from build123d import *

# Parameters (mm, degrees)
BOSS_EXTRUDE1_DEPTH       = 30
BOSS_EXTRUDE2_DEPTH       = 105
FILLET1_R                 = 5
CONVERT_SOLID2_START      = -80
CONVERT_SOLID2_DEPTH      = 160
SKETCH12_R                = 7
SKETCH12_R_2              = 2.5
AXLE_HOLES_DEPTH          = 141.121375957
SKETCH13_W                = 39.25
SKETCH13_H                = 43.333333333
SKETCH13_H_2              = 43.333333334
WEIGHT_SAVING_HOLES_DEPTH = 2
CHAMFER1_SIZE             = 5
M3_START                  = -52.5
M3_CLEARANCE_SLOT1_DEPTH  = 105
M2_CLEARANCE_HOLE1_D      = 2.4


# Read off the part's stored shape, not the designer's step: Convert-Solid2, M3 Clearance Slot1
with BuildPart() as part:
    # Sketch1 → Boss-Extrude1 (new body)
    with BuildSketch(Plane(origin=(0, 0, 0), x_dir=(1, 0, 0), z_dir=(0, 1, 0))):
        Polygon((-52.5, -80), (0, -80), (52.5, -80), (52.5, 80), (-52.5, 80), align=None)
    extrude(amount=BOSS_EXTRUDE1_DEPTH)

    # Sketch11 → Boss-Extrude2 (add)
    with BuildSketch(Plane(origin=(52.5, 0, 0), x_dir=(0, 0, -1), z_dir=(1, 0, 0))):
        with BuildLine():
            Line((-18.091022132, 30), (-15.974774553, 35.814342437))
            ThreePointArc((-15.974774553, 35.814342437), (0, 47), (15.974774553, 35.814342437))
            Line((15.974774553, 35.814342437), (18.091022132, 30))
            Line((18.091022132, 30), (-18.091022132, 30))
        make_face()
    extrude(amount=-BOSS_EXTRUDE2_DEPTH)

    # Fillet1
    fillet1_edges = [part.edges().sort_by_distance(p)[0] for p in [
        (0, 30, -18.091022132),
        (0, 30, 18.091022132),
    ]]
    fillet(fillet1_edges, radius=FILLET1_R)

    # Convert-Solid2 outline → Convert-Solid2 (cut)
    with BuildSketch(Plane.XY.offset(CONVERT_SOLID2_START)):
        with BuildLine():
            Line((-54, 5.2e-08), (-49.5, 0))
            ThreePointArc((-49.5, 0), (-51.621320344, 0.878679656), (-52.5, 3))
            Line((-52.5, 3), (-52.499999977, 48))
            Line((-52.499999977, 48), (-54, 48))
            Line((-54, 48), (-54, 5.2e-08))
        make_face()
        with BuildLine():
            ThreePointArc((52.5, 3), (51.621320344, 0.878679656), (49.5, 0))
            Line((49.5, 0), (54, 5.2e-08))
            Line((54, 5.2e-08), (54, 48))
            Line((54, 48), (52.499999977, 48))
            Line((52.499999977, 48), (52.5, 3))
        make_face()
        with BuildLine():
            Line((50.5, 3), (50.5, 48))
            Line((50.5, 48), (-50.5, 48))
            Line((-50.5, 48), (-50.5, 3))
            ThreePointArc((-50.5, 3), (-50.207106781, 2.292893219), (-49.5, 2))
            Line((-49.5, 2), (49.5, 2))
            ThreePointArc((49.5, 2), (50.207106781, 2.292893219), (50.5, 3))
        make_face()
    extrude(amount=CONVERT_SOLID2_DEPTH, mode=Mode.SUBTRACT)

    # Sketch12 → Axle Holes (cut, through all)
    with BuildSketch(Plane(origin=(52.5, 0, 0), x_dir=(0, 0, -1), z_dir=(1, 0, 0))):
        with Locations((0, 30)):
            Circle(SKETCH12_R)
        with Locations((35, 15)):
            Circle(SKETCH12_R_2)
        with BuildLine():
            Line((-35, 19.5), (-25, 19.5))
            ThreePointArc((-25, 19.5), (-22, 16.5), (-25, 13.5))
            Line((-25, 13.5), (-35, 13.5))
            ThreePointArc((-35, 13.5), (-38, 16.5), (-35, 19.5))
        make_face()
    extrude(amount=-AXLE_HOLES_DEPTH, mode=Mode.SUBTRACT)

    # Sketch13 → Weight Saving Holes (cut)
    with BuildSketch(Plane(origin=(0, 2, 0), x_dir=(1, 0, 0), z_dir=(0, 1, 0))):
        with Locations((-23.375, 50.833333334)):
            Rectangle(SKETCH13_W, SKETCH13_H)
        with Locations((-23.375, 0)):
            Rectangle(SKETCH13_W, SKETCH13_H_2)
        with Locations((-23.375, -50.833333334)):
            Rectangle(SKETCH13_W, SKETCH13_H)
        with Locations((23.375, -50.833333334)):
            Rectangle(SKETCH13_W, SKETCH13_H)
        with Locations((23.375, 0)):
            Rectangle(SKETCH13_W, SKETCH13_H_2)
        with Locations((23.375, 50.833333334)):
            Rectangle(SKETCH13_W, SKETCH13_H)
    extrude(amount=-WEIGHT_SAVING_HOLES_DEPTH, mode=Mode.SUBTRACT)

    # Chamfer1
    chamfer1_edges = [part.edges().sort_by_distance(p)[0] for p in [
        (43, 1, -72.5),
        (3.75, 1, -72.5),
        (3.75, 1, -29.166666667),
        (43, 1, -29.166666667),
        (43, 1, -21.666666667),
        (3.75, 1, -21.666666667),
        (3.75, 1, 21.666666667),
        (43, 1, 21.666666667),
        (43, 1, 29.166666667),
        (3.75, 1, 29.166666667),
        (3.75, 1, 72.5),
        (43, 1, 72.5),
        (-43, 1, 29.166666667),
        (-43, 1, 72.5),
        (-3.75, 1, 72.5),
        (-3.75, 1, 29.166666667),
        (-43, 1, -21.666666667),
        (-43, 1, 21.666666667),
        (-3.75, 1, 21.666666667),
        (-3.75, 1, -21.666666667),
        (-43, 1, -72.5),
        (-43, 1, -29.166666667),
        (-3.75, 1, -29.166666667),
        (-3.75, 1, -72.5),
    ]]
    chamfer(chamfer1_edges, length=CHAMFER1_SIZE)

    # M3 Clearance Slot1 outline → M3 Clearance Slot1 (cut)
    with BuildSketch(Plane.YZ.offset(M3_START)):
        with BuildLine():
            ThreePointArc((12.080710415, 26.033343618), (10.380710415, 27.733343618), (8.680710415, 26.033343618))
            Line((8.680710415, 26.033343618), (8.680710415, 19.433343618))
            ThreePointArc((8.680710415, 19.433343618), (10.380710415, 17.733343618), (12.080710415, 19.433343618))
            Line((12.080710415, 19.433343618), (12.080710415, 26.033343618))
        make_face()
        with BuildLine():
            ThreePointArc((12.080710415, 38.453085966), (10.380710415, 40.153085966), (8.680710415, 38.453085966))
            Line((8.680710415, 38.453085966), (8.680710415, 31.853085966))
            ThreePointArc((8.680710415, 31.853085966), (10.380710415, 30.153085966), (12.080710415, 31.853085966))
            Line((12.080710415, 31.853085966), (12.080710415, 38.453085966))
        make_face()
        with BuildLine():
            ThreePointArc((24.319289585, 40.566656382), (22.619289585, 42.266656382), (20.919289585, 40.566656382))
            Line((20.919289585, 40.566656382), (20.919289585, 33.966656382))
            ThreePointArc((20.919289585, 33.966656382), (22.619289585, 32.266656382), (24.319289585, 33.966656382))
            Line((24.319289585, 33.966656382), (24.319289585, 40.566656382))
        make_face()
        with BuildLine():
            ThreePointArc((24.319289585, 28.146914034), (22.619289585, 29.846914034), (20.919289585, 28.146914034))
            Line((20.919289585, 28.146914034), (20.919289585, 21.546914034))
            ThreePointArc((20.919289585, 21.546914034), (22.619289585, 19.846914034), (24.319289585, 21.546914034))
            Line((24.319289585, 21.546914034), (24.319289585, 28.146914034))
        make_face()
    extrude(amount=M3_CLEARANCE_SLOT1_DEPTH, mode=Mode.SUBTRACT)

    # M2 Clearance Hole1 (through all)
    with Locations(Plane.ZY.offset(52.5)):
        with Locations((-35, 20), (-30, 15), (-35, 10), (-40, 15)):
            Hole(M2_CLEARANCE_HOLE1_D / 2)


solid = part.part
CAD build for the part. Positions are in the model's coordinates, mm. A direction names the side the tool comes from. Round coordinates to 2 decimals unless told otherwise and drop trailing zeros. Order: outer loops, then holes, each group sorted by start corner. A loop starts at its lowest first (then second) coordinate and runs counter-clockwise, first axis right, second up. Notation, with made-up numbers: (50.25, 79) -> (76.25, 79) arc R17 ccw to (76.25, 110) -> close; hole circle Ø6 at (48, -14.75). An arc over 180 degrees is marked (long way). Write item = value, one per line. Start each with the question number.
(1) Pin check, flat tips, straight feed: P1, Ø4.5, axis at y = 15, z = -35, coming from the +X side; P2, Ø1.6, axis at y = 0.5, z = -57.5, coming from the +X side; P3, Ø2, axis at x = 51.5, z = 24.5, coming from the -Y side; P4, Ø2, axis at y = 0.5, z = -50, coming from the -X side. Stop position of each tip, or through.
(2) Pull direction Z, two halves, no side cores. Call faces 6 (the flat face through (-52.5, 20, -1)), 7 (the cylindrical face through (-51.51, 30.88, -18.76)), 8 (the flat face through (-6.215, 1.014, 19.132)): released by +Z, released by -Z, zero draft, split by the parting line, or undercut.
(3) Cut at B-B, the plane x = -40. List the corners of the cut face in (y, z), then the cut area to 3 significant figures.
(4) Cut at A-A, the plane x = -23. List the corners of the cut face in (y, z), then the cut area to 3 significant figures.
(5) Which spindle directions (+Z, -Z, +X, -X, +Y, -Y) get a long thin tool onto all of the face, cutting with end or side? Do faces 1 (the flat face through (50.5, 20, -1)), 2 (the cylindrical face through (51.64, 0.9, -1.12)), 3 (the flat face through (-40.535, 1.014, 31.702)), 4 (the flat face through (52.5, 20, 1)), 5 (the cylindrical face through (-51.5, 16.6, 22)). Say none if no direction does.
(6) Probe line 1 (X direction, y = 4.5, z = -6.5); line 2 (Y direction, x = -51.7, z = -35); line 3 (Y direction, x = -45, z = 55). List the from-to ranges inside material, lowest first. Write a range as [from, to].
Model answer:
q1.P1 = through
q1.P2 = 51.97
q1.P3 = 0.17
q1.P4 = -52.1
q2.face_6 = zero draft
q2.face_7 = released by -Z
q2.face_8 = undercut
q3.outline = (0, -80) -> (2, -80) -> (2, -70.5) -> (0, -70.5) -> close; (0, -31.17) -> (2, -31.17) -> (2, -19.67) -> (0, -19.67) -> close; (0, 19.67) -> (2, 19.67) -> (2, 31.17) -> (0, 31.17) -> close; (0, 70.5) -> (2, 70.5) -> (2, 80) -> (0, 80) -> close
q3.area = 84.0 mm2
q4.outline = (0, -80) -> (2, -80) -> (2, -72.5) -> (0, -72.5) -> close; (0, -29.17) -> (2, -29.17) -> (2, -21.67) -> (0, -21.67) -> close; (0, 21.67) -> (2, 21.67) -> (2, 29.17) -> (0, 29.17) -> close; (0, 72.5) -> (2, 72.5) -> (2, 80) -> (0, 80) -> close
q4.area = 60.0 mm2
q5.face_1 = +Z, -Z, +Y
q5.face_2 = +Z, -Z, +X, -Y
q5.face_3 = +Y, -Y
q5.face_4 = +Z, -Z, +X, +Y, -Y
q5.face_5 = +X, -X
q6.line_1 = [-52.5, -50.5], [50.5, 52.5]
q6.line_2 = [0.96, 8.8], [11.2, 12.5], [17.5, 18.8], [21.2, 30]
q6.line_3 = [0, 2]
